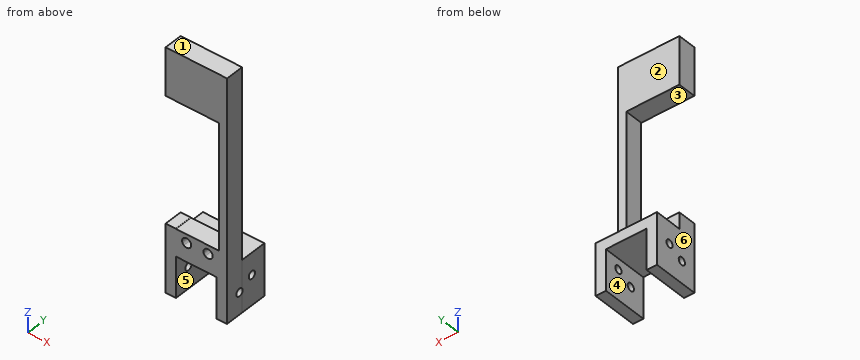
Autodesk Inventor part; units mm, degrees
ref_plane "Work Plane1" through (0, 0, 0) normal (0, 0, 1) x (1, 0, 0)
ref_plane "Work Plane2" through (0, 0, 0) normal (0, 0, 1) x (1, 0, 0)
ref_plane "YZ Plane" through (0, 0, 0) normal (1, 0, 0) x (0, 1, 0)
ref_plane "Work Plane1" through (0, 0, 0) normal (0, 0, 1) x (1, 0, 0)
ref_plane "Work Plane2" through (0, 0, 0) normal (0, 0, 1) x (1, 0, 0)
sketch "Sketch2" plane through (0, 0, 0) normal (0, 0, 1) x (1, 0, 0)
  line L0 (0, 0) -> (19.05, 0)
  line L1 (19.05, 0) -> (19.05, 431.8) construction
  line L2 (0, 431.8) -> (19.05, 431.8)
  line L3 (0, 0) -> (0, 431.8) construction
  line L4 (18.5, 323.6774) -> (1.5, 323.6774)
  line L5 (18.5, 323.6774) -> (19.1476, 323.6774)
  line L6 (1.5, 323.6774) -> (0, 323.6774)
  line L7 (-4.8174, 323.6774) -> (23.8674, 323.6774)
  line L8 (23.8674, 323.6774) -> (23.8674, 332.1879)
  line L9 (23.8674, 332.1879) -> (-4.8174, 332.1879)
  line L10 (-4.8174, 332.1879) -> (-4.8174, 323.6774)
  line L11 (9.525, 431.8) -> (9.525, 312.4258) construction
  line L12 (9.525, 327.9326) -> (-4.8174, 327.9326) construction
  line L13 (23.8674, 327.9326) -> (9.525, 327.9326) construction
extrude "Extrusion1" add sketch "Sketch2" along normal blind 61.9125
sketch "Sketch3" plane through (-4.8174, 323.6774, 0) normal (0, -1, 0) x (1, 0, 0)
  arc A0 (8.4674, 58.3733) -> (11.1674, 58.3733) centre (9.8174, 56.7) ccw
  arc A1 (18.4674, 58.3733) -> (21.1674, 58.3733) centre (19.8174, 56.7) ccw
  arc A2 (11.1674, 7.0267) -> (8.4674, 7.0267) centre (9.8174, 8.7) ccw
  arc A3 (21.1674, 7.0267) -> (18.4674, 7.0267) centre (19.8174, 8.7) ccw
  circle A4 centre (9.8174, 8.7) radius 2.15
  circle A5 centre (19.8174, 8.7) radius 2.15
  circle A6 centre (9.8174, 56.7) radius 2.15
  circle A7 centre (19.8174, 56.7) radius 2.15
  point P0 (4.8174, 0)
extrude "Extrusion2" cut sketch "Sketch3" against normal through all
sketch "Sketch4" plane through (-4.8174, 332.1879, 0) normal (0, 1, 0) x (1, 0, 0)
  line L0 (4.8174, -14.2) -> (4.8174, -51.2)
  line L1 (6.3174, -52.7) -> (23.3174, -52.7)
  line L2 (24.8174, -51.2) -> (24.8174, -14.2)
  line L3 (23.3174, -12.7) -> (6.3174, -12.7)
  line L4 (4.8174, -52.7) -> (24.8174, -52.7)
  line L5 (24.8174, -52.7) -> (24.8174, -12.7)
  line L6 (24.8174, -12.7) -> (4.8174, -12.7)
  line L7 (4.8174, -12.7) -> (4.8174, -52.7)
  point P0 (4.8174, 0)
extrude "Extrusion3" cut sketch "Sketch4" against normal through all
sketch "Sketch6" plane through (0, 0, 0) normal (0, 0, -1) x (-1, 0, 0)
  line L0 (4.8174, 323.6774) -> (-23.8674, 323.6774)
  line L1 (4.8174, 332.1879) -> (4.8174, 323.6774)
  line L2 (-23.8674, 332.1879) -> (4.8174, 332.1879)
  line L3 (-23.8674, 323.6774) -> (-23.8674, 332.1879)
  point P0 (0, 0)
extrude "Extrusion4" add sketch "Sketch6" along normal blind 19.05
sketch "Sketch7" plane through (-4.8174, 332.1879, 61.9125) normal (0, 1, 0) x (1, 0, 0)
  line L0 (4.8174, 70.6755) -> (4.8174, 80.9625)
  line L1 (4.8174, 61.9125) -> (4.8174, 70.6755)
  line L2 (23.8674, 61.9125) -> (23.8674, 70.6755)
  line L3 (23.8674, 71.4375) -> (23.8674, 80.9625)
  line L4 (23.8674, 61.9125) -> (4.8174, 61.9125)
  line L5 (4.8174, 61.9125) -> (4.8174, 80.9625)
  line L6 (4.8174, 80.9625) -> (23.8674, 80.9625)
  line L7 (23.8674, 80.9625) -> (23.8674, 61.9125)
extrude "Extrusion5" cut sketch "Sketch7" against normal through all
sketch "Sketch8" plane through (-4.8174, 332.1879, 61.9125) normal (0, 1, 0) x (1, 0, 0)
  line L0 (28.6847, 80.9625) -> (28.6847, 0)
  line L1 (0, 80.9625) -> (0, 0)
  line L2 (4.8174, 61.9125) -> (4.8174, 80.9625)
  line L3 (0, 80.9625) -> (4.8174, 80.9625)
  line L4 (0, 80.9625) -> (0, 0)
  line L5 (28.6847, 0) -> (0, 0)
  line L6 (28.6847, 80.9625) -> (28.6847, 0)
  line L7 (23.8674, 80.9625) -> (28.6847, 80.9625)
  line L8 (23.8674, 80.9625) -> (23.8674, 61.9125)
  line L9 (23.8674, 61.9125) -> (4.8174, 61.9125)
  line L10 (24.8174, 49.2125) -> (24.8174, 9.2125)
  line L11 (24.8174, 9.2125) -> (4.8174, 9.2125)
  line L12 (4.8174, 9.2125) -> (4.8174, 49.2125)
  line L13 (4.8174, 49.2125) -> (24.8174, 49.2125)
  circle A0 centre (9.8174, 5.2125) radius 2.15
  circle A1 centre (9.8174, 53.2125) radius 2.15
  circle A2 centre (19.8174, 53.2125) radius 2.15
  circle A3 centre (19.8174, 5.2125) radius 2.15
  line L14 (28.6847, 56.7746) -> (0, 56.7746)
  line L15 (28.6847, 56.7746) -> (57.3695, 56.7746) construction
  point P0 (4.8174, 61.9125)
  dimension "d10" = 180
extrude "Extrusion6" add sketch "Sketch8" along normal blind 12.7 contours L0 L14 L1 L3 L2 L9 L8 L7
sketch "Sketch10" plane through (23.8674, 323.6774, 61.9125) normal (1, 0, 0) x (0, 0, -1)
  point P0 (61.9125, -323.6774)
sketch "Sketch11" plane through (-4.8174, 323.6774, 61.9125) normal (-1, 0, 0) x (0, 0, 1)
  line L0 (0, 0) -> (-80.9625, 0)
  line L1 (0, 8.5105) -> (0, 0)
  line L2 (-56.7746, 8.5105) -> (0, 8.5105)
  line L3 (-56.7746, 8.5105) -> (-56.7746, 21.2105)
  line L4 (-80.9625, 21.2105) -> (-56.7746, 21.2105)
  line L5 (-80.9625, 0) -> (-80.9625, 21.2105)
  circle A0 centre (-66.9806, 14.1192) radius 1.7859
  circle A1 centre (-70.7565, 7.0913) radius 1.7859
  line L6 (-66.9806, 14.1192) -> (-66.9806, 21.2105) construction
  line L7 (-70.7565, 7.0913) -> (-70.7565, 0) construction
  line L8 (-80.9625, 0) -> (0, 0) construction
  line L9 (-70.7565, 7.0913) -> (-80.9625, 7.0913) construction
  line L10 (-80.9625, 0) -> (-80.9625, 21.2105) construction
  line L11 (-66.9806, 14.1192) -> (-56.7746, 14.1192) construction
  point P0 (-61.9125, -323.6774)
  dimension "d13" = 3.5719
  dimension "d14" = 3.5719
extrude "Extrusion7" cut sketch "Sketch11" against normal through all contours A0 | A1
sketch "Sketch12" plane through (-4.8174, 332.1879, 61.9125) normal (0, 1, 0) x (1, 0, 0)
  point P0 (4.8174, 61.9125)
move faces "Move1" translate (0, 0, 31.75) faces at (4.7442, 329.3511, 61.9125)
delete faces "Delete1" heal yes whole lump no faces at (6.978, 329.3511, 57.5427) (17.143, 329.3511, 56.527)
move faces "Move2" translate (0, 0, 18.6486) faces at (6.6667, 329.3511, 52.7)
sketch "Sketch13" plane through (-4.8174, 323.6774, 93.6625) normal (0, -1, 0) x (1, 0, 0)
  line L0 (0, -88.5246) -> (0, 0)
  line L1 (4.8174, -22.3139) -> (0, -22.3139)
  line L2 (0, -22.3139) -> (0, -80.9198)
  line L3 (0, -80.9198) -> (4.8174, -80.9198)
  line L4 (4.8174, -80.9198) -> (4.8174, -22.3139)
  point P0 (4.8174, -93.6625)
extrude "Extrusion8" cut sketch "Sketch13" against normal through all
sketch "Sketch14" plane through (-4.8174, 323.6774, 93.6625) normal (0, -1, 0) x (1, 0, 0)
  line L0 (9.8174, -84.9625) -> (9.8174, -14.9173) construction
  line L1 (19.8174, -84.9625) -> (19.8174, -14.9173) construction
  circle A0 centre (19.8174, -84.9625) radius 2.15
  circle A1 centre (19.8174, -84.9625) radius 2.15
  circle A2 centre (19.8174, -14.9173) radius 1.7859
  circle A3 centre (9.8174, -14.9173) radius 1.7859
  circle A4 centre (19.8174, -84.9625) radius 1.7859
  circle A5 centre (9.8174, -84.9625) radius 1.7859
  point P0 (4.8174, -93.6625)
  dimension "d29" = 3.5719
  dimension "d30" = 3.5719
  dimension "d31" = 3.5719
  dimension "d32" = 3.5719
properties part number "servo mount"
Verification items for the finished model (mm, model axes). Face numbers are marked on the shaded views. A direction names the side the tool comes from. Coordinates: 2 decimals unless noted, no trailing zeros. Write each loop counter-clockwise with the first axis right and the second up, starting at its lowest first coordinate (ties: lowest second). Pieces come first, ordered by that corner, then holes. Notation, with made-up numbers: M 49,42.5 L 93,42.5 A23 ccw 93,79.5 Z; hole C 9.5,34.25 d8. An arc over 180 degrees is marked long. Use CSV: the item, a comma, the result in double quotes.
Q1. Mould release check, pull along X, two halves, no side actions. Record for the marked faces 5 and 6: pulls with the +X half, pulls with the -X half, needs draft (parallel to the pull), parting line crosses it, or undercut.
Computed values:
face 5,"undercut"
face 6,"pulls with the -X half"
Q2. Set-up check for the marked faces 1, 2, 3 and 4: record each of +Z, -Z, +X, -X, +Y, -Y from which the full face is reachable in a straight line by a thin tool's end or side.
Computed values:
face 1,"+Z, +X, -X, +Y, -Y"
face 2,"+Z, +X, -X, +Y"
face 3,"-X, +Y, -Y"
face 4,"-Z, +Y, -Y"
Q3. Section check A-A, the plane x = 15. Enter the section's corners in (y, z), and give its area (3 significant figures).
Computed values:
outline,"M 323.68,0 L 344.89,0 L 344.89,5.14 L 332.19,5.14 L 332.19,6.55 L 323.68,6.55 Z; M 323.68,10.85 L 332.19,10.85 L 332.19,12.7 L 323.68,12.7 Z; M 323.68,71.35 L 332.19,71.35 L 332.19,93.66 L 323.68,93.66 Z"
area,"327 mm²"
Q4. Section check B-B, the plane z = 8.7. Enter the section's corners in (x, y).
Computed values:
outline,"M -4.82,323.68 L 2.85,323.68 L 2.85,332.19 L -4.82,332.19 Z; M 7.15,323.68 L 12.85,323.68 L 12.85,332.19 L 7.15,332.19 Z; M 17.15,323.68 L 23.87,323.68 L 23.87,332.19 L 17.15,332.19 Z"
Q5. Section check D-D, the plane y = 325.75. Enter the section's corners in (x, z).
Computed values:
outline,"M -4.82,-19.05 L 0,-19.05 L 0,0 L 19.05,0 L 19.05,-19.05 L 23.87,-19.05 L 23.87,93.66 L -4.82,93.66 L -4.82,71.35 L 20,71.35 L 20,12.7 L 0,12.7 L 0,12.74 L -4.82,12.74 Z; hole C 5,8.7 d4.3; hole C 15,8.7 d4.3"
Q6. Go/stop test with flat-tipped pins: P1, Ø2.5, axis at x = 3, y = 326, coming from the -Z side; P2, Ø2, axis at y = 330.77, z = -8.84, coming from the -X side; P3, Ø12, axis at y = 331.5, z = 36, coming from the -X side; P4, Ø1, axis at x = 15.5, y = 334.5, coming from the +Z side. Record where each tip stops, or that it passes through.
Computed values:
P1,"z = 0"
P2,"through"
P3,"x = 20"
P4,"z = 5.14"
Q7. Section check C-C, the plane y = 342.5. Enter the section's corners in (x, z), and give its area (3 significant figures).
Computed values:
outline,"M -4.82,-19.05 L 0,-19.05 L 0,0 L 19.05,0 L 19.05,-19.05 L 23.87,-19.05 L 23.87,5.14 L -4.82,5.14 Z"
area,"331 mm²"
Q8. Thickness scan on line 1 along X through (y, z) = (325.5, 8.7); line 2 along Z through (x, y) = (11.5, 330); line 3 along X through (y, z) = (329, 7.5). Record the ranges inside material, lowest first. Write a range as [from, to].
Computed values:
line 1,"[-4.82, 2.85], [7.15, 12.85], [17.15, 23.87]"
line 2,"[0, 12.7], [71.35, 93.66]"
line 3,"[-4.82, 3.22], [6.78, 13.22], [16.78, 23.87]"
